```python
from build123d import *

# Parameters (mm, degrees)
ESQUISSE2_W             = 177.5
ESQUISSE2_H             = 20
BOSS_EXTRU_1_DEPTH      = 20
BOSS_EXTRU_3_DEPTH      = 110
ESQUISSE5_W             = 10
ESQUISSE5_H             = 10
BOSS_EXTRU_4_DEPTH      = 30
D_GAGEMENT_M31_D        = 3.2
D_GAGEMENT_M31_DEPTH    = 10
D_GAGEMENT_M31_TIP      = 0.96137699
ESQUISSE8_W             = 15
ESQUISSE8_H             = 15
ENL_V_MAT_EXTRU_1_DEPTH = 60


with BuildPart() as part:
    # Esquisse2 → Boss.-Extru.1 (new body)
    with BuildSketch(Plane(origin=(0, 0, 0), x_dir=(1, 0, 0), z_dir=(0, 1, 0))):
        with Locations((88.75, 10)):
            Rectangle(ESQUISSE2_W, ESQUISSE2_H)
    extrude(amount=BOSS_EXTRU_1_DEPTH)

    # Esquisse4 → Boss.-Extru.3 (add)
    with BuildSketch(Plane(origin=(0, 20, 0), x_dir=(1, 0, 0), z_dir=(0, 1, 0))):
        Polygon((0, 20), (20, 20), (26.229306319, 0), (0, 0), align=None)
    extrude(amount=BOSS_EXTRU_3_DEPTH)

    # Esquisse5 → Boss.-Extru.4 (add)
    with BuildSketch(Plane(origin=(177.5, 0, 0), x_dir=(0, 0, -1), z_dir=(1, 0, 0))):
        with Locations((10, 10)):
            Rectangle(ESQUISSE5_W, ESQUISSE5_H)
    extrude(amount=BOSS_EXTRU_4_DEPTH)

    # Dégagement M31
    with Locations(Plane(origin=(10, 80, -20), x_dir=(-1, 0, 0), z_dir=(0, 0, -1))):
        with Locations((0, 0)):
            Hole(D_GAGEMENT_M31_D / 2, depth=D_GAGEMENT_M31_DEPTH)
            with Locations((0, 0, -(D_GAGEMENT_M31_DEPTH + D_GAGEMENT_M31_TIP / 2))):  # 118° drill point
                Cone(0, D_GAGEMENT_M31_D / 2, D_GAGEMENT_M31_TIP, mode=Mode.SUBTRACT)

    # Esquisse8 → Enlèv. mat.-Extru.1 (cut)
    with BuildSketch(Plane(origin=(0, 130, 0), x_dir=(1, 0, 0), z_dir=(0, 1, 0))):
        with Locations((10, 10)):
            Rectangle(ESQUISSE8_W, ESQUISSE8_H)
    extrude(amount=-ENL_V_MAT_EXTRU_1_DEPTH, mode=Mode.SUBTRACT)


solid = part.part
```
Source: CAD feature listing. Evaluate the final solid. Frame: model axes, mm. A direction names the side the tool comes from. Give positions to 0.01 mm unless a question says otherwise; leave off trailing zeros. Write each loop counter-clockwise with the first axis right and the second up, starting at its lowest first coordinate (ties: lowest second). Pieces come first, ordered by that corner, then holes.
1. Section query C-C (x = 102). Return the cut outline in (y, z).
2. Section query B-B (z = -8). Return the cut outline in (x, y), then the cut area to 3 significant figures.
3. First-contact query: pin 1 (11 mm diameter, centred on x = 193.5, z = -10.5, fed in from -Y); pin 2 (12 mm diameter, centred on y = 100.5, z = -13, fed in from +X); pin 3 (5 mm diameter, centred on x = 195.5, y = 11, fed in from +Z); pin 4 (4 mm diameter, centred on x = 111.5, z = -4, fed in from -Y). Flat tips, straight axial feed; report the tip coordinate or a pass-through.
4. Pull-direction query (X, two-part tool) for faces 4 (the face through (55, 17, -20)), 5 (the face through (207.5, 10, -10)), 6 (the face through (10, 100, -2.5)); classes: +X half, -X half, draft (parallel to the pull), parting line (faces both ways), or undercut.
5. Material intervals for line 1 along Y through (x, z) = (10, -18.05); line 2 along Z through (x, y) = (16.5, 86); line 3 along Y through (x, z) = (40.5, -4.75), sorted ascending.
6. Access query for faces 1 (the face through (10, 100, -17.5)), 2 (the face through (192, 15, -10)), 3 (the face through (23.07, 74.23, -10.14)). Directions: +Z, -Z, +X, -X, +Y, -Y. A direction counts if a zero-diameter tool reaches every point of the face in a straight line with its end or side. Return the directions, or none.
7. Section query D-D (y = 28). Return the cut outline in (x, z), then the cut area to 3 significant figures.
8. Section query A-A (y = 98). Return the cut outline in (x, z).
Output values:
1. outline: (0, -20) - (20, -20) - (20, 0) - (0, 0) - close
2. outline: (0, 0) - (177.5, 0) - (177.5, 5) - (207.5, 5) - (207.5, 15) - (177.5, 15) - (177.5, 20) - (23.74, 20) - (23.74, 130) - (17.5, 130) - (17.5, 70) - (2.5, 70) - (2.5, 130) - (0, 130) - close
2. area: 5,560 mm2
3. pin 1: stops at y = 5
3. pin 2: stops at x = 24.05
3. pin 3: stops at z = -5
3. pin 4: stops at y = 0
4. face 4: draft
4. face 5: +X half
4. face 6: undercut
5. line 1: y = 0 to 78.4, 81.6 to 130
5. line 2: z = -20 to -17.5, -2.5 to 0
5. line 3: y = 0 to 20
6. face 1: +Y
6. face 2: +Z, -Z, +X, +Y
6. face 3: -Z, +X, +Y
7. outline: (0, -20) - (20, -20) - (26.23, 0) - (0, 0) - close
7. area: 462 mm2
8. outline: (0, -20) - (20, -20) - (26.23, 0) - (0, 0) - close; hole (2.5, -17.5) - (17.5, -17.5) - (17.5, -2.5) - (2.5, -2.5) - close
